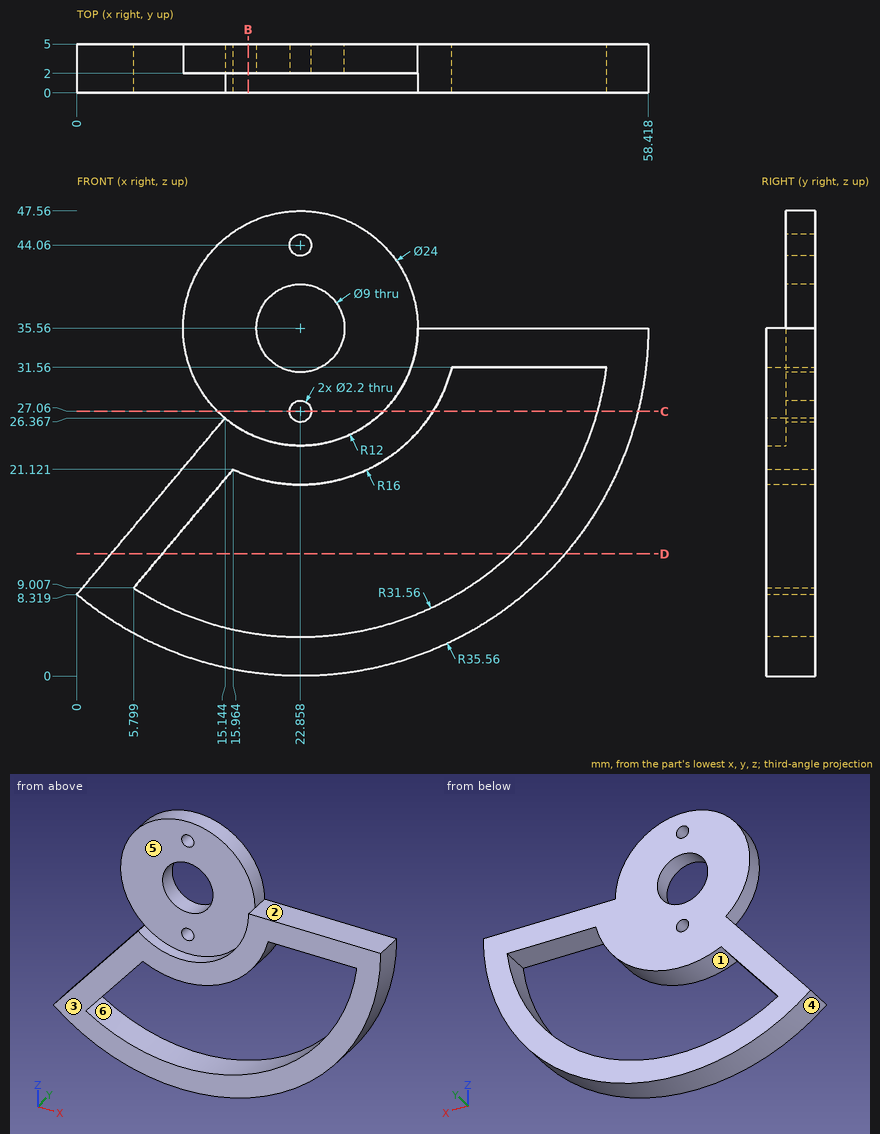
Geometry: see drawing. Coordinates: mm, zero at the bounding-box minimum. A direction names the side the tool comes from. Give positions to 0.01 mm unless a question says otherwise; leave off trailing zeros. Order: outer loops, then holes, each group sorted by start corner. A loop starts at its lowest first (then second) coordinate and runs counter-clockwise, first axis right, second up.
1. Cut plane C-C (z = 27.06). Return loops of the section in (x, y).
Computed:
outline: (14.39, 2) - (21.76, 2) - (21.76, 5) - (14.39, 5) - close; (23.96, 2) - (31.33, 2) - (31.33, 0) - (36.41, 0) - (36.41, 5) - (23.96, 5) - close; (53.25, 0) - (57.39, 0) - (57.39, 5) - (53.25, 5) - close
2. Set-up query: the marked faces 1, 2 and 3. Return all of +Z, -Z, +X, -X, +Y, -Y with unobstructed straight access to the full face (end or side cutting, diameter ignored); none if empty.
Computed:
face 1: +Y, -Y
face 2: +Z, +X, +Y, -Y
face 3: +Z, -Z, +X, -X, -Y
3. Draft query along Z for the marked faces 4, 5 and 6. Return one class per face: released by +Z, released by -Z, zero draft, split by the parting line, or undercut.
Computed:
face 4: released by -Z
face 5: zero draft
face 6: undercut
4. Cut plane D-D (z = 12.5). Return loops of the section in (x, y) (1 decimal).
Computed:
outline: (3.5, 0) - (8.7, 0) - (8.7, 5) - (3.5, 5) - close; (44.4, 0) - (49.9, 0) - (49.9, 5) - (44.4, 5) - close
5. Cut plane B-B (x = 17.5). Return loops of the section in (y, z) (1 decimal).
Computed:
outline: (0, 0.4) - (5, 0.4) - (5, 4.5) - (0, 4.5) - close; (0, 20.5) - (5, 20.5) - (5, 46.3) - (2, 46.3) - (2, 24.8) - (0, 24.8) - close
6. Line query: probe 1 along X at (y, z) = (3.7, 35); probe 2 along Z at (x, y) = (46, 1.75); probe 3 along X at (y, z) = (4.6, 24) (1 decimal). Output: solid intervals per line, ascending.
Computed:
probe 1: x = 10.87 to 18.39, 27.32 to 58.41
probe 2: z = 8.56 to 14.1, 31.56 to 35.56
probe 3: x = 13.2 to 33.9, 52.2 to 56.5
7. Pin query (flat end, axial travel): pin 1 Ø4 at (x, z) = (32, 41) entering from -Y; pin 2 Ø5.5 at (x, z) = (22.86, 35.56) entering from -Y; pin 3 Ø1.5 at (x, y) = (18, 3) entering from +Z (1 decimal); pin 4 Ø1 at (y, z) = (2, 40.5) entering from +X (1 decimal). Return the tip coordinate at first contact, or that it passes through.
Computed:
pin 1: stops at y = 2
pin 2: passes through
pin 3: stops at z = 46.8
pin 4: stops at x = 34
